Verification items for the finished model (mm, model axes). A direction names the side the tool comes from. Give positions to 0.01 mm unless a question says otherwise; leave off trailing zeros. Write each loop counter-clockwise with the first axis right and the second up, starting at its lowest first coordinate (ties: lowest second). Pieces come first, ordered by that corner, then holes. Notation, with made-up numbers: (19, 84) - (47, 84) arc R10 cw to (47, 95) - close; hole circle Ø4 at (24.25, 89). An arc over 180 degrees is marked (long way). Put each result on its own line as item: value.
from build123d import *

# Parameters (mm, degrees)
SKETCH1_R           = 2.465
BOSS_EXTRUDE1_DEPTH = 2.9
SKETCH2_R           = 1.45
BOSS_EXTRUDE2_DEPTH = 16
CUT_EXTRUDE1_DEPTH  = 1.9
CHAMFER1_SIZE       = 0.25


with BuildPart() as part:
    # Sketch1 → Boss-Extrude1 (new body)
    with BuildSketch(Plane(origin=(0, 0, 0), x_dir=(1, 0, 0), z_dir=(0, 1, 0))):
        Circle(SKETCH1_R)
    extrude(amount=BOSS_EXTRUDE1_DEPTH)

    # Sketch2 → Boss-Extrude2 (add)
    with BuildSketch(Plane(origin=(0, 2.9, 0), x_dir=(1, 0, 0), z_dir=(0, 1, 0))):
        Circle(SKETCH2_R)
    extrude(amount=BOSS_EXTRUDE2_DEPTH)

    # Sketch3 → Cut-Extrude1 (cut)
    with BuildSketch(Plane.XZ):
        Polygon((0.733234842, -1.27), (1.466469684, 0), (0.733234842, 1.27), (-0.733234842, 1.27), (-1.466469684, 0), (-0.733234842, -1.27), align=None)
    extrude(amount=-CUT_EXTRUDE1_DEPTH, mode=Mode.SUBTRACT)

    # Chamfer1
    chamfer1_edges = [part.edges().sort_by_distance(p)[0] for p in [
        (-1.45, 18.9, 0),
    ]]
    chamfer(chamfer1_edges, length=CHAMFER1_SIZE)


solid = part.part
Q1. Section check A-A, the plane x = 0. Record the cut outline in (y, z) (3 decimals).
Answers follow:
outline: (0, -2.465) - (2.9, -2.465) - (2.9, -1.45) - (18.65, -1.45) - (18.9, -1.2) - (18.9, 1.2) - (18.65, 1.45) - (2.9, 1.45) - (2.9, 2.465) - (0, 2.465) - (0, 1.27) - (1.9, 1.27) - (1.9, -1.27) - (0, -1.27) - close
Q2. Scan lines: line 1 along Y through (x, z) = (1.4, -0.9); line 2 along X through (y, z) = (10, 0.7); line 3 along Y through (x, z) = (-0.85, 0.1). Record each from-to range of solid material in increasing order.
Answers follow:
line 1: y = 0 to 2.9
line 2: x = -1.27 to 1.27
line 3: y = 1.9 to 18.9
Q3. Set-up check for faces 1 (the face through (0, 1.9, 0)), 2 (the face through (0, 2.9, 2)), 3 (the face through (-1.956, 1.43, 1.5)): record each of +Z, -Z, +X, -X, +Y, -Y from which the full face is reachable in a straight line by a thin tool's end or side.
Answers follow:
face 1: -Y
face 2: +Y
face 3: +Y, -Y
Q4. Release check for a two-part mould opening along X. For faces 4 (the face through (-1.45, 10.66, -0.06)), 5 (the face through (1.1, 0, 1.1)), 6 (the face through (1.105, 0.937, 0.626)) record: released by +X, released by -X, zero draft, split by the parting line, or undercut.
Answers follow:
face 4: split by the parting line
face 5: zero draft
face 6: undercut
Q5. Section check B-B, the plane y = 11.5. Record the cut outline in (x, z), plus the area to 3 significant figures.
Answers follow:
outline: circle Ø2.9 at (0, 0)
area: 6.61 mm2
Q6. Go/stop test with a flat-tipped pin: pin 1 Ø1 at (x, y) = (0.5, 9) entering from +Z. Record where the tip stops, or that it passes through.
Answers follow:
pin 1: stops at z = 1.45
Q7. Section check C-C, the plane x = -2.1. Record the cut outline in (y, z), plus the area to 3 significant figures.
Answers follow:
outline: (0, -1.29) - (2.9, -1.29) - (2.9, 1.29) - (0, 1.29) - close
area: 7.49 mm2
